Geometry: see drawing. Coordinates: mm, zero at the bounding-box minimum. Round coordinates to 2 decimals unless told otherwise and drop trailing zeros. Write each loop counter-clockwise with the first axis right and the second up, starting at its lowest first coordinate (ties: lowest second). Pieces come first, ordered by that corner, then holes. Notation, with made-up numbers: M 89,72 L 107,72 A20 cw 107,101 Z; hole C -34,-37.75 d2. An arc over 180 degrees is marked long. Use one line per item in the form item = value. Start each with the question number.
Item 1: Pull-direction query (X, two-part tool) for the marked faces 1, 2 and 3; classes: pulls with the +X half, pulls with the -X half, needs draft (parallel to the pull), parting line crosses it, or undercut.
Item 2: Section query D-D (x = 12.25). Return loops of the section in (y, z), and give its area (3 significant figures).
Item 3: Section query A-A (y = 7). Return loops of the section in (x, z).
Item 4: Section query C-C (z = 1.75). Return loops of the section in (x, y), and give its area (3 significant figures).
Item 5: Ray query, probe 1 along Y at (x, z) = (7, 16); probe 2 along Y at (x, z) = (6, 9.25); probe 3 along X at (y, z) = (8.5, 13.75). Return the intervals inside material, ascending.
Item 6: Pin query (flat end, axial travel): pin 1 Ø6 at (x, z) = (10.5, 16) entering from +Y; pin 2 Ø2 at (y, z) = (12, 15.5) entering from -X; pin 3 Ø5 at (x, z) = (10, 19.5) entering from -Y. Return the tip coordinate at first contact, or that it passes through.
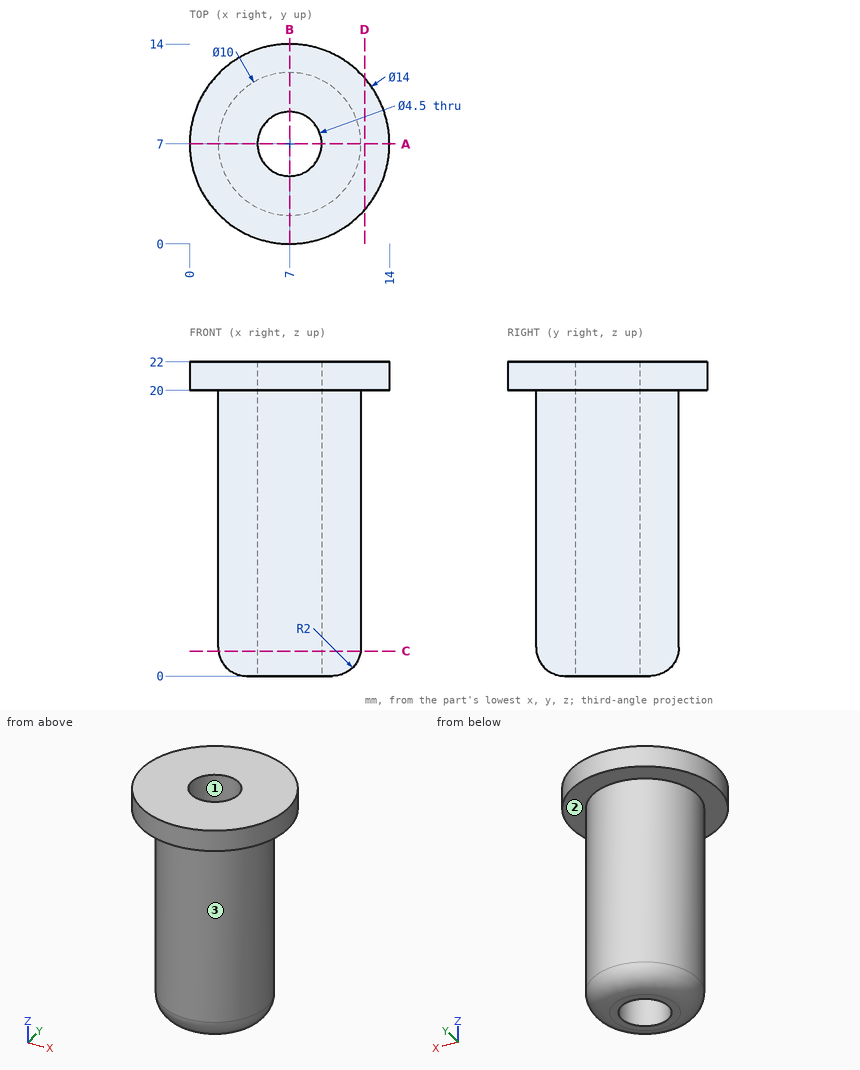
Working result:
q1.face_1 = undercut
q1.face_2 = needs draft
q1.face_3 = parting line crosses it
q2.outline = M 2.37,20 L 11.63,20 L 11.63,22 L 2.37,22 Z
q2.area = 18.5 mm²
q3.outline = M 0,20 L 2,20 L 2,2 A2 ccw 4,0 L 4.75,0 L 4.75,22 L 0,22 Z; M 9.25,0 L 10,0 A2 ccw 12,2 L 12,20 L 14,20 L 14,22 L 9.25,22 Z
q4.outline = C 7,7 d9.97; hole C 7,7 d4.5
q4.area = 62.1 mm²
q5.probe_1 = 2 to 4.75, 9.25 to 12
q5.probe_2 = 2.1 to 4.98, 9.02 to 11.9
q5.probe_3 = 2.23 to 5.32, 8.68 to 11.77
q6.pin_1 = 11.97
q6.pin_2 = 4
q6.pin_3 = 0.02
